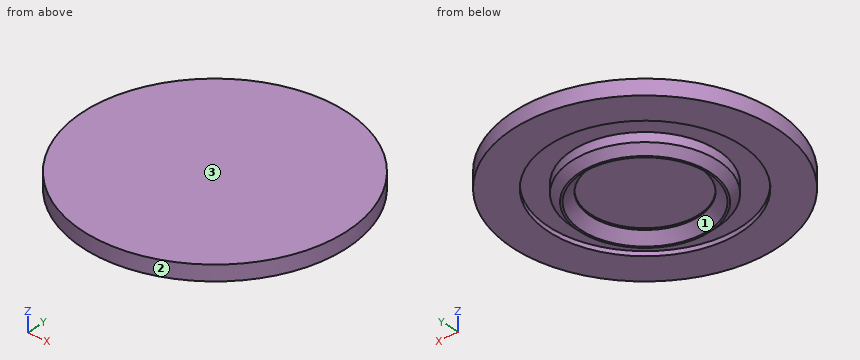
Autodesk Inventor part; units mm, degrees
ref_plane "YZ Plane" through (0, 0, 0) normal (1, 0, 0) x (0, 1, 0)
ref_plane "XZ Plane" through (0, 0, 0) normal (0, 1, 0) x (-1, 0, 0)
ref_plane "XY Plane" through (0, 0, 0) normal (0, 0, 1) x (1, 0, 0)
sketch "Skizze1" plane through (0, 0, 0) normal (1, 0, 0) x (0, 1, 0)
  line L0 (-20.6011, -1.9989) -> (-21.4, -1.2)
  line L1 (-21.4, -1.2) -> (-21.4, 0)
  line L2 (-25, 0) -> (-25, -0.6)
  line L3 (-22.8485, -0.6) -> (-20.8497, -2.5989)
  line L4 (0.345, -0.6) -> (5, -0.6)
  line L5 (5, -0.6) -> (5, 1.4)
  line L6 (-12.5, -6.6891) -> (-12.5, -2.8)
  line L7 (5, 1.4) -> (-12.155, 1.4)
  line L8 (-6.155, -0.8) -> (-6.155, -1) construction
  line L9 (-6.155, -1) -> (-18.155, -1) construction
  line L10 (-18.155, -1) -> (-18.155, -0.8) construction
  line L11 (-18.155, -0.8) -> (-13.2371, -0.918) construction
  line L12 (-12.155, 1.4) -> (-12.155, -0.7885)
  line L13 (-5.1181, -0.7885) -> (-5.1181, -1) construction
  line L14 (-5.1181, -0.7885) -> (-5.1181, -1) construction
  line L15 (-5.1181, -0.7885) -> (-5.1181, -1)
  line L16 (-6.155, -1) -> (-6.5167, -1)
  line L17 (-5.7914, -1.4086) -> (-6.1109, -1.0891)
  line L18 (-3.6, 0) -> (0, 0)
  line L19 (-5.7914, -1.4086) -> (-6.1109, -1.0891)
  line L20 (-19.1918, -1) -> (-5.1181, -1)
  line L21 (-5.1181, -0.7885) -> (-12.155, -0.7885)
  line L22 (-5.1181, -1) -> (-3.9212, -2.2)
  line L23 (-3.6692, -2.2) -> (-2.6692, -1.2) construction
  line L24 (-3.9212, -2.2) -> (-3.6692, -2.2)
  line L25 (-3.6692, -2.2) -> (-2.6692, -1.2)
  line L26 (-2.6692, -1.2) -> (-2.6692, 0)
  line L27 (0.345, 0) -> (0.345, -0.6) construction
  line L28 (0.345, -0.6) -> (0.345, 0)
  line L29 (0.345, 0) -> (-2.6692, 0)
  point P0 (0, -0.6)
  point P1 (-2.1515, -0.6)
  point P2 (-20.8023, -2.2)
  point P3 (-22.8485, -0.6)
  point P4 (-21.0508, -2.8)
  point P5 (-12.155, -1)
  point P6 (-5, -2.2)
  point P7 (-3.2, 0)
  dimension "d1" = 2
revolve "Umdrehung1" add sketch "Skizze1" angle 360 about axis through (0, -12.155, 1.4) along (0, 0, -1)
properties part number "50_ETL_Membrane_Mould_Lower_v0"
Part model, mm, in its own coordinate system. Face numbers are marked on the shaded views. Coordinates: 2 decimals unless noted, no trailing zeros. Order: outer loops, then holes, each group sorted by start corner. A loop starts at its lowest first (then second) coordinate and runs counter-clockwise, first axis right, second up. Notation, with made-up numbers: (-17.5, 30) - (1.5, 30) arc R20 cw to (1.5, 52) - close; hole circle Ø7 at (80, 19.5). An arc over 180 degrees is marked (long way). Return JSON: item names as keys, results as strings. Group by question number.
Item 1: Cut at B-B (y = -26). List the corners of the cut face in (x, z).
Item 2: Cut at D-D (x = -11). List the corners of the cut face in (y, z), plus the area to 3 significant figures.
Item 3: Pin check, flat tips, straight feed: pin 1 (15.5 mm diameter, centred on x = 0, y = -10.5, fed in from -Z); pin 2 (8.5 mm diameter, centred on x = 0, y = -12.155, fed in from -Z); pin 3 (2 mm diameter, centred on x = -6, z = 0, fed in from +Y). Stop position of each tip, or through.
Item 4: Drill centre lines: probe 1 along X at (y, z) = (-5.5, -0.3); probe 2 along Y at (x, z) = (-2, -0.3); probe 3 along Z at (x, y) = (3, -10.5). Where is each one in solid material? Low to high. Write a range as from..to.
Item 5: Pull direction X, two halves, no side cores. Call the marked faces 1, 2 and 3: pulls with the +X half, pulls with the -X half, needs draft (parallel to the pull), parting line crosses it, or undercut.
Item 6: Cut at C-C (x = 10). List the corners of the cut face in (y, z) (3 decimals), plus the area to 3 significant figures.
Check values:
{
 "1": {"outline": "(-10.13, -0.6) - (10.13, -0.6) - (10.13, 1.4) - (-10.13, 1.4) - close"},
 "2": {"outline": "(-25.32, -0.6) - (-18.09, -0.6) - (-18.09, 0) - (-6.22, 0) - (-6.22, -0.6) - (1.01, -0.6) - (1.01, 1.4) - (-25.32, 1.4) - close", "area": "45.5 mm2"},
 "3": {"pin 1": "stops at z = -2.2", "pin 2": "stops at z = -0.79", "pin 3": "stops at y = 4.26"},
 "4": {"probe 1": "x = -15.81..-10.58, -6.76..6.76, 10.58..15.81", "probe 2": "y = -29.19..-24.49, -21.43..-2.88, 0.18..4.88", "probe 3": "z = -0.79..1.4"},
 "5": {"face 1": "undercut", "face 2": "parting line crosses it", "face 3": "needs draft"},
 "6": {"outline": "(-26.094, -0.6) - (-19.655, -0.6) - (-19.655, 0) - (-4.655, 0) - (-4.655, -0.6) - (1.784, -0.6) - (1.784, 1.4) - (-26.094, 1.4) - close", "area": "46.8 mm2"}
}
